Verification items for the finished model (mm, model axes). Round coordinates to 2 decimals unless told otherwise and drop trailing zeros. Order: outer loops, then holes, each group sorted by start corner. A loop starts at its lowest first (then second) coordinate and runs counter-clockwise, first axis right, second up. Notation, with made-up numbers: (87.5, -19.75) -> (101.5, -19.75) arc R17 cw to (101.5, 1.25) -> close; hole circle Ø3 at (73.5, 38). An arc over 180 degrees is marked (long way). Return JSON: item names as keys, results as strings. Group by question number.
1) Depth check by flat-ended pin: pin 1 (1.5 mm diameter, centred on x = 99, z = 2, fed in from +Y); pin 2 (1.5 mm diameter, centred on y = -17, z = 2, fed in from +X); pin 3 (0.9 mm diameter, centred on y = 49, z = 1, fed in from -X). Enter the tip coordinate at first touch or a pass-through.
2) Section check C-C on x = -65. Enter the section's corners in (y, z), plus the area to 3 significant figures.
3) Section check D-D on y = 24. Enter the section's corners in (x, z).
4) Section check B-B on y = -2. Enter the section's corners in (x, z).
5) Section check A-A on y = -22. Enter the section's corners in (x, z), plus the area to 3 significant figures.
6) Scan lines: L1, parallel to X at y = 8.5, z = 0.2; L2, parallel to X at y = 11, z = 1.4; L3, parallel to Y at x = 9.5, z = 1.3. Record each from-to range of solid material in increasing order.
```python
from build123d import *

# Parameters (mm, degrees)
BOSS_EXTRUDE1_DEPTH = 3
SKETCH2_W           = 3
SKETCH2_H           = 20
SKETCH2_W_2         = 40
SKETCH2_H_2         = 3
CUT_EXTRUDE1_DEPTH  = 3


with BuildPart() as part:
    # Sketch1 → Boss-Extrude1 (new body)
    with BuildSketch(Plane.XY):
        Polygon((-60, 5.09773753), (-60, -50), (-70, -50), (-70, -47), (-90, -47), (-90, -50), (-100, -50), (-100, 50), (100, 50), (100, -50), (90, -50), (90, -47), (70, -47), (70, -50), (60, -50), (60, -40.178411678), (60, 20), (-60, 20), align=None)
    extrude(amount=BOSS_EXTRUDE1_DEPTH)

    # Sketch2 → Cut-Extrude1 (cut)
    with BuildSketch(Plane.XY.offset(3)):
        with Locations((-98.5, -20)):
            Rectangle(SKETCH2_W, SKETCH2_H)
        with Locations((-98.5, 20)):
            Rectangle(SKETCH2_W, SKETCH2_H)
        with Locations((0, 48.5)):
            Rectangle(SKETCH2_W_2, SKETCH2_H_2)
        with Locations((80, 48.5)):
            Rectangle(SKETCH2_W_2, SKETCH2_H_2)
        with Locations((98.5, 20)):
            Rectangle(SKETCH2_W, SKETCH2_H)
        with Locations((98.5, -20)):
            Rectangle(SKETCH2_W, SKETCH2_H)
        with Locations((-80, 48.5)):
            Rectangle(SKETCH2_W_2, SKETCH2_H_2)
    extrude(amount=-CUT_EXTRUDE1_DEPTH, mode=Mode.SUBTRACT)


solid = part.part
```
Check result:
{
 "1": {"pin 1": "y = 47", "pin 2": "x = 97", "pin 3": "x = -60"},
 "2": {"outline": "(-50, 0) -> (47, 0) -> (47, 3) -> (-50, 3) -> close", "area": "291 mm^2"},
 "3": {"outline": "(-97, 0) -> (97, 0) -> (97, 3) -> (-97, 3) -> close"},
 "4": {"outline": "(-100, 0) -> (-60, 0) -> (-60, 3) -> (-100, 3) -> close; (60, 0) -> (100, 0) -> (100, 3) -> (60, 3) -> close"},
 "5": {"outline": "(-97, 0) -> (-60, 0) -> (-60, 3) -> (-97, 3) -> close; (60, 0) -> (97, 0) -> (97, 3) -> (60, 3) -> close", "area": "222 mm^2"},
 "6": {"L1": "-100 to -60, 60 to 100", "L2": "-97 to -60, 60 to 97", "L3": "20 to 47"}
}
